from build123d import *
from build123d.topology import SkipClean

# Parameters (mm, degrees)
CROQUIS1_W              = 60
CROQUIS1_H              = 40
CROQUIS1_R              = 1.5
SALIENTE_EXTRUIR1_DEPTH = 17.96
SALIENTE_EXTRUIR2_START = 4.7625
CROQUIS3_W              = 15
CROQUIS3_H              = 40
CROQUIS3_R              = 1.5
SALIENTE_EXTRUIR2_DEPTH = 4.7625
CROQUIS4_R              = 7.75
SALIENTE_EXTRUIR3_DEPTH = 4.7625
REDONDEO2_R             = 10
CORTAR_EXTRUIR1_DEPTH   = 5
CROQUIS6_W              = 10
CROQUIS6_H              = 40
CORTAR_EXTRUIR2_DEPTH   = 7
CORTAR_EXTRUIR3_START   = -8
CROQUIS7_W              = 30
CROQUIS7_H              = 40
CROQUIS7_R              = 7.75
CORTAR_EXTRUIR3_DEPTH   = 8


with BuildPart() as part:
    # Croquis1 → Saliente-Extruir1 (new body)
    with BuildSketch(Plane(origin=(0, 0, 0), x_dir=(0, 0, -1), z_dir=(1, 0, 0))):
        Rectangle(CROQUIS1_W, CROQUIS1_H)
        with Locations((-25, 15)):
            Circle(CROQUIS1_R, mode=Mode.SUBTRACT)
        with Locations(Location((25, 15, 0), (0, 0, 180))):
            Circle(CROQUIS1_R, mode=Mode.SUBTRACT)
        with Locations((25, -15)):
            Circle(CROQUIS1_R, mode=Mode.SUBTRACT)
        with Locations(Location((-25, -15, 0), (0, 0, 180))):
            Circle(CROQUIS1_R, mode=Mode.SUBTRACT)
    extrude(amount=SALIENTE_EXTRUIR1_DEPTH)

    # Croquis3 → Saliente-Extruir2 (add)
    # profile 1 of 2: a face of its own
    with SkipClean():  # the faces are left unmerged after this step: merging them gives an invalid solid
        with BuildSketch(Plane.ZY.offset(SALIENTE_EXTRUIR2_START)):
            with Locations((-22.5, 0)):
                Rectangle(CROQUIS3_W, CROQUIS3_H)
            with Locations((-25, -15)):
                Circle(CROQUIS3_R, mode=Mode.SUBTRACT)
            with Locations((-25, 15)):
                Circle(CROQUIS3_R, mode=Mode.SUBTRACT)
        # profile 2 of 2: a face of its own
        with BuildSketch(Plane.ZY.offset(SALIENTE_EXTRUIR2_START)):
            with Locations((22.5, 0)):
                Rectangle(CROQUIS3_W, CROQUIS3_H)
            with Locations((25, -15)):
                Circle(CROQUIS3_R, mode=Mode.SUBTRACT)
            with Locations((25, 15)):
                Circle(CROQUIS3_R, mode=Mode.SUBTRACT)
        extrude(amount=-SALIENTE_EXTRUIR2_DEPTH)

    # Croquis4 → Saliente-Extruir3 (add)
    with SkipClean():  # the faces are left unmerged after this step: merging them gives an invalid solid
        with BuildSketch(Plane.ZY):
            with Locations(Location((0, 0, 0), (0, 0, 180))):
                Circle(CROQUIS4_R)
        extrude(amount=SALIENTE_EXTRUIR3_DEPTH)

    # Redondeo2
    # the kernel refuses this fillet: 10 mm, written as the material it takes off along each edge
    with BuildSketch(Plane(origin=(17.96, -45, -30), x_dir=(-1, 0, 0), z_dir=(0, 1, 0)), Plane(origin=(17.96, 45, 30), x_dir=(-1, 0, 0), z_dir=(0, -1, 0))) as redondeo2_piece_1:
        with BuildLine():
            CenterArc((REDONDEO2_R, REDONDEO2_R), REDONDEO2_R, 180, 90)
            Line((0, REDONDEO2_R), (0, 0))
            Line((0, 0), (REDONDEO2_R, 0))
        make_face()
    extrude(amount=90, mode=Mode.SUBTRACT)
    with BuildSketch(Plane(origin=(17.96, 20, -55), x_dir=(0, -1, 0), z_dir=(0, 0, 1))) as redondeo2_piece_2:
        with BuildLine():
            CenterArc((REDONDEO2_R, -REDONDEO2_R), REDONDEO2_R, 90, 90)
            Line((0, -REDONDEO2_R), (0, 0))
            Line((0, 0), (REDONDEO2_R, 0))
        make_face()
    extrude(amount=110, mode=Mode.SUBTRACT)
    with BuildSketch(Plane(origin=(17.96, -20, 55), x_dir=(-1, 0, 0), z_dir=(0, 0, -1))) as redondeo2_piece_3:
        with BuildLine():
            CenterArc((REDONDEO2_R, REDONDEO2_R), REDONDEO2_R, 180, 90)
            Line((0, REDONDEO2_R), (0, 0))
            Line((0, 0), (REDONDEO2_R, 0))
        make_face()
    extrude(amount=110, mode=Mode.SUBTRACT)

    # Croquis5 → Cortar-Extruir1 (cut)
    with BuildSketch(Plane(origin=(17.96, 0, 0), x_dir=(0, 0, -1), z_dir=(1, 0, 0))):
        Polygon((-25, 18.464101615), (-28, 16.732050808), (-28, 13.267949192), (-25, 11.535898385), (-22, 13.267949192), (-22, 16.732050808), align=None)
        Polygon((25, 18.464101615), (22, 16.732050808), (22, 13.267949192), (25, 11.535898385), (28, 13.267949192), (28, 16.732050808), align=None)
        Polygon((25, -18.464101615), (28, -16.732050808), (28, -13.267949192), (25, -11.535898385), (22, -13.267949192), (22, -16.732050808), align=None)
        Polygon((-25, -18.464101615), (-22, -16.732050808), (-22, -13.267949192), (-25, -11.535898385), (-28, -13.267949192), (-28, -16.732050808), align=None)
    extrude(amount=-CORTAR_EXTRUIR1_DEPTH, mode=Mode.SUBTRACT)

    # Croquis6 → Cortar-Extruir2 (cut)
    with BuildSketch(Plane.ZY.offset(4.7625)):
        with Locations((25, 0)):
            Rectangle(CROQUIS6_W, CROQUIS6_H)
        with Locations((-25, 0)):
            Rectangle(CROQUIS6_W, CROQUIS6_H)
    extrude(amount=-CORTAR_EXTRUIR2_DEPTH, mode=Mode.SUBTRACT)

    # Croquis7 → Cortar-Extruir3 (cut)
    with BuildSketch(Plane.ZY.offset(CORTAR_EXTRUIR3_START)):
        Rectangle(CROQUIS7_W, CROQUIS7_H)
        with Locations(Location((0, 0, 0), (0, 0, 180))):
            Circle(CROQUIS7_R, mode=Mode.SUBTRACT)
    extrude(amount=CORTAR_EXTRUIR3_DEPTH, mode=Mode.SUBTRACT)


solid = part.part
The listing builds one solid part. Answer for the finished solid, in the listing's coordinates (mm). A direction names the side the tool comes from. Give positions to 0.01 mm unless a question says otherwise; leave off trailing zeros. Write each loop counter-clockwise with the first axis right and the second up, starting at its lowest first coordinate (ties: lowest second). Pieces come first, ordered by that corner, then holes.
1) Section D-D (z = 0) is taken. Write down the section's boundary in (x, y).
2) Find the intervals of material crossed by L1, parallel to Y at x = 7.25, z = 25; L2, parallel to Y at x = 10.25, z = -25; L3, parallel to Z at x = -2.25, y = -16, in increasing order.
3) Section C-C (y = 0) is taken. Write down the section's boundary in (x, z).
4) For a pull along Y with two mould halves and no side action, classify faces 1 (the face through (13.908, 17.394, 23.146)), 2 (the face through (3, -20, -21)), 3 (the face through (3, 20, 21)) as pulls with the +Y half, pulls with the -Y half, needs draft (parallel to the pull), parting line crosses it, or undercut.
5) Section A-A (x = 3.75) is taken. Write down the section's boundary in (y, z).
6) Given P1, Ø2, axis at y = -12.5, z = -21.5, coming from the -X side; P2, Ø3, axis at x = 16, y = 14.5, coming from the +Z side; P3, Ø0.8, axis at x = 13.5, y = 15, coming from the -Z side, each flat-ended and moving along its own axis, determine where each tip first touches the part or whether it passes through.
7) A tool of negligible diameter and unlimited length cuts with its end or side. For faces 4 (the face through (-1, 0, -20)), 5 (the face through (12.96, -16.5, 25.7)), 6 (the face through (5, 0, -30)), from which of +Z, -Z, +X, -X, +Y, -Y can it reach the whole face along a straight path? Write none if from no direction.
8) Section B-B (y = -15) is taken. Write down the section's boundary in (x, z).
Response:
1. outline: (-4.76, -7.75) - (8, -7.75) - (8, -20) arc R10 ccw to (17.96, -10) - (17.96, 10) arc R10 ccw to (8, 20) - (8, 7.75) - (-4.76, 7.75) - close
2. L1: y = -20 to -16.5, -13.5 to 13.5, 16.5 to 20
2. L2: y = -19.73 to -16.5, -13.5 to 13.5, 16.5 to 19.73
2. L3: z = -20 to -15, 15 to 20
3. outline: (-4.76, -20) - (2.24, -20) - (2.24, -30) - (7.96, -30) arc R10 ccw to (17.96, -20) - (17.96, 20) arc R10 ccw to (7.96, 30) - (2.24, 30) - (2.24, 20) - (-4.76, 20) - (-4.76, 15) - (8, 15) - (8, 7.75) - (-4.76, 7.75) - (-4.76, -7.75) - (8, -7.75) - (8, -15) - (-4.76, -15) - close
4. face 1: undercut
4. face 2: pulls with the -Y half
4. face 3: pulls with the +Y half
5. outline: (-20, -30) - (20, -30) - (20, -15) - (-20, -15) - close; (-20, 15) - (20, 15) - (20, 30) - (-20, 30) - close; circle Ø15.5 at (0, 0); hole circle Ø3 at (-15, -25); hole circle Ø3 at (-15, 25); hole circle Ø3 at (15, -25); hole circle Ø3 at (15, 25)
6. P1: stops at x = 2.24
6. P2: stops at z = 22.46
6. P3: stops at z = -28.58
7. face 4: -Z, -X, +Y, -Y
7. face 5: +X
7. face 6: -Z, +X, -X, +Y, -Y
8. outline: (-4.76, -20) - (2.24, -20) - (2.24, -23.5) - (12.96, -23.5) - (12.96, -22) - (16.62, -22) - (16.62, 22) - (12.96, 22) - (12.96, 23.5) - (2.24, 23.5) - (2.24, 20) - (-4.76, 20) - (-4.76, 15) - (8, 15) - (8, -15) - (-4.76, -15) - close; (2.24, -30) - (7.96, -30) arc R10 ccw to (13.96, -28) - (12.96, -28) - (12.96, -26.5) - (2.24, -26.5) - close; (2.24, 26.5) - (12.96, 26.5) - (12.96, 28) - (13.96, 28) arc R10 ccw to (7.96, 30) - (2.24, 30) - close
